CAD build for the part. Positions are in the model's coordinates, mm. Give positions to 0.01 mm unless a question says otherwise; leave off trailing zeros. Write each loop counter-clockwise with the first axis right and the second up, starting at its lowest first coordinate (ties: lowest second). Pieces come first, ordered by that corner, then holes. Notation, with made-up numbers: (3, 5.5) -> (13, 5.5) arc R17 cw to (13, 20.5) -> close; hole circle Ø11 at (-3.75, -1). An arc over 180 degrees is marked (long way). Answer as a JSON object with one key per item and string values.
```python
from build123d import *

# Parameters (mm, degrees)
F0_W     = 50.8
F0_H     = 50.8
F1_DEPTH = 25.4
F3_DEPTH = 50.8
F4_SIZE  = 6.35
F5_R     = 6.35
F6_DEPTH = 50.801


with BuildPart() as f1:
    # F0 (on Front) → F1 (new body, symmetric)
    with BuildSketch(Plane.XZ):
        Rectangle(F0_W, F0_H)
    extrude(amount=F1_DEPTH, both=True)

    # F2 (on face) → F3 (cut)
    with BuildSketch(Plane.XY.offset(25.4)):
        with BuildLine():
            ThreePointArc((-25.4, -23.5464301965), (-13.8644325812, -14.1990316571), (-9.525, 0))
            ThreePointArc((-9.525, 0), (-13.8644325812, 14.1990316571), (-25.4, 23.5464301965))
            Line((-25.4, 23.5464301965), (-25.4, -23.5464301965))
        make_face()
    extrude(amount=-F3_DEPTH, mode=Mode.SUBTRACT)

    # F4
    f4_edges = [f1.edges().sort_by_distance(p)[0] for p in [
        (25.4, -25.4, 0),
        (25.4, 25.4, 0),
    ]]
    chamfer(f4_edges, length=F4_SIZE)

    # F5 (on face) → F6 (cut, through all)
    with BuildSketch(Plane.XZ.offset(25.4)):
        with Locations((6.35, 0)):
            Circle(F5_R)
    extrude(amount=-F6_DEPTH, mode=Mode.SUBTRACT)


solid = f1.part
```
1) Mould opens along Z. For faces 1 (the flat face through (5, 0, 25.4)), 2 (the flat face through (5, 0, -25.4)), 3 (the flat face through (-25.4, 24, 0)), 4 (the cylindrical face through (12.216, -0.356, -2.432)) say: released by +Z, released by -Z, zero draft, split by the parting line, or undercut.
Model answer:
{"face 1": "released by +Z", "face 2": "released by -Z", "face 3": "zero draft", "face 4": "undercut"}
2) Slice it at B-B (z = 0). List the corners of the cut face in (x, y) (3 decimals), then the cut area to 3 significant figures.
Model answer:
{"outline": "(-25.4, -25.4) -> (0, -25.4) -> (0, 25.4) -> (-25.4, 25.4) -> (-25.4, 23.546) arc R25.4 cw to (-25.4, -23.546) -> close; (12.7, -25.4) -> (19.05, -25.4) -> (25.4, -19.05) -> (25.4, 19.05) -> (19.05, 25.4) -> (12.7, 25.4) -> close", "area": "1,350 mm2"}
3) Slice it at A-A (x = 6.35). List the corners of the cut face in (y, z).
Model answer:
{"outline": "(-25.4, -25.4) -> (25.4, -25.4) -> (25.4, -6.35) -> (-25.4, -6.35) -> close; (-25.4, 6.35) -> (25.4, 6.35) -> (25.4, 25.4) -> (-25.4, 25.4) -> close"}
4) Slice it at D-D (z = -8.5). List the corners of the cut face in (x, y) (3 decimals), then the cut area to 3 significant figures.
Model answer:
{"outline": "(-25.4, -25.4) -> (19.05, -25.4) -> (25.4, -19.05) -> (25.4, 19.05) -> (19.05, 25.4) -> (-25.4, 25.4) -> (-25.4, 23.546) arc R25.4 cw to (-25.4, -23.546) -> close", "area": "2,000 mm2"}
5) Wall check: probe 1 along Z at (x, y) = (6.35, -1.5); probe 2 along X at (y, z) = (8, -1); probe 3 along Y at (x, z) = (-15, 13). Give the ranges that are in metal, low to high.
Model answer:
{"probe 1": "z = -25.4 to -6.35, 6.35 to 25.4", "probe 2": "x = -10.82 to 0.08, 12.62 to 25.4", "probe 3": "y = -25.4 to -15.75, 15.75 to 25.4"}
6) Slice it at C-C (y = 13). List the corners of the cut face in (x, z).
Model answer:
{"outline": "(-13.1, -25.4) -> (25.4, -25.4) -> (25.4, 25.4) -> (-13.1, 25.4) -> close; hole circle Ø12.7 at (6.35, 0)"}
7) Pin check, flat tip, straight feed: pin 1 (4 mm diameter, centred on y = -19.5, z = 8.5, fed in from -X). Stop position of the tip, or through.
Model answer:
{"pin 1": "stops at x = -21.4"}
